The model under review builds one solid part; all positions refer to its coordinate system, in mm. Face numbers are marked on the shaded views. A direction names the side the tool comes from. Coordinates: 2 decimals unless noted, no trailing zeros. Write each loop counter-clockwise with the first axis right and the second up, starting at its lowest first coordinate (ties: lowest second). Pieces come first, ordered by that corner, then holes.
1) Add section A-A, the plane x = -8.5. State the section outline as (y, z) points.
2) For P1, Ø4, axis at x = 2.93, z = -7.36, coming from the +Y side; P2, Ø4, axis at x = -7.5, y = 6, coming from the +Z side; P3, Ø2, axis at x = -25, z = 10, coming from the +Y side; P4, Ø2, axis at x = -27.07, z = 22.64, coming from the -Y side, all flat-tipped, find the tip position at first contact; note any pin that passes through.
3) Add section C-C, the plane y = 1.5. State the section outline as (x, z) points.
4) For line 1 (Z direction, x = -21, y = 9.25); line 2 (Y direction, x = -29, z = 24); line 3 (Y direction, x = -18.5, z = 6), list the stretches that pass through material, from the lowest coordinate up.
5) Machinability: for the marked faces 1, 2, 3, 4 and 5, which of the approach directions +Z, -Z, +X, -X, +Y, -Y give a long, thin tool a straight path to every point of the face, cutting with its end or side? Answer none if there is none.
6) Add section D-D, the plane y = 13.25. State the section outline as (x, z) points.
7) Add section B-B, the plane x = -1.5. State the section outline as (y, z) points, then the cut area to 3 significant figures.
8) Mouldability with a two-part tool opening along Z and no side actions: class the marked faces 6, 7 and 8 as released by +Z, released by -Z, zero draft, split by the parting line, or undercut.
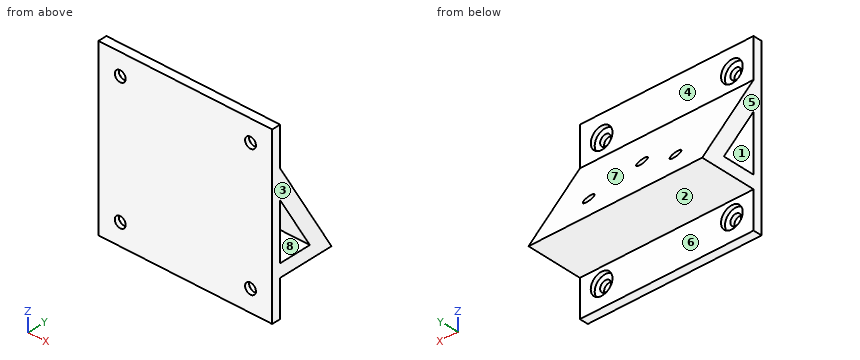
from build123d import *

# Parameters (mm, degrees)
SKETCH1_W           = 40
SKETCH1_H           = 40
BOSS_EXTRUDE1_DEPTH = 2
SKETCH2_R           = 1.25
CUT_EXTRUDE1_DEPTH  = 3
BOSS_EXTRUDE2_DEPTH = 40
SKETCH5_R           = 2.5
CUT_EXTRUDE3_DEPTH  = 1
CUT_EXTRUDE4_DEPTH  = 41
CUT_EXTRUDE5_REACH  = 19.232
SKETCH6_R           = 1.25
SKETCH11_R          = 2.6
CUT_EXTRUDE6_DEPTH  = 1.2


with BuildPart() as part:
    # Sketch1 → Boss-Extrude1 (new body)
    with BuildSketch(Plane(origin=(0, 0, 0), x_dir=(1, 0, 0), z_dir=(0, 1, 0))):
        with Locations((-12.069207341, -7.637914169)):
            Rectangle(SKETCH1_W, SKETCH1_H)
    extrude(amount=BOSS_EXTRUDE1_DEPTH)

    # Sketch2 → Cut-Extrude1 (cut, through all)
    with BuildSketch(Plane(origin=(0, 2, 0), x_dir=(1, 0, 0), z_dir=(0, 1, 0))):
        with Locations((-27.069207341, -22.637914169)):
            Circle(SKETCH2_R)
        with Locations((-27.069207341, 7.362085831)):
            Circle(SKETCH2_R)
        with Locations((2.930792659, 7.362085831)):
            Circle(SKETCH2_R)
        with Locations((2.930792659, -22.637914169)):
            Circle(SKETCH2_R)
    extrude(amount=-CUT_EXTRUDE1_DEPTH, mode=Mode.SUBTRACT)

    # Sketch4 → Boss-Extrude2 (add)
    with BuildSketch(Plane(origin=(7.930792659, 0, 0), x_dir=(0, 0, -1), z_dir=(1, 0, 0))):
        Polygon((-18.637914169, 2), (3.878746329, 2), (3.878746329, 15), align=None)
    extrude(amount=-BOSS_EXTRUDE2_DEPTH)

    # Sketch5 → Cut-Extrude3 (cut)
    with BuildSketch(Plane(origin=(0, 2, 0), x_dir=(1, 0, 0), z_dir=(0, 1, 0))):
        with Locations((2.930792659, 7.362085831)):
            Circle(SKETCH5_R)
        with Locations((2.930792659, -22.637914169)):
            Circle(SKETCH5_R)
        with Locations((37.902040206, 5.850032714)):
            Circle(SKETCH5_R)
        with Locations((-27.069207341, 7.362085831)):
            Circle(SKETCH5_R)
        with Locations((-27.069207341, -22.637914169)):
            Circle(SKETCH5_R)
    extrude(amount=-CUT_EXTRUDE3_DEPTH, mode=Mode.SUBTRACT)

    # Sketch9 → Cut-Extrude4 (cut, through all)
    with BuildSketch(Plane(origin=(7.930792659, 0, 0), x_dir=(0, 0, -1), z_dir=(1, 0, 0))):
        Polygon((-12.121253671, 2), (0.878746329, 2), (0.878746329, 9.505553499), align=None)
    extrude(amount=-CUT_EXTRUDE4_DEPTH, mode=Mode.SUBTRACT)

    # Sketch6 → Cut-Extrude5 (cut, up to next)
    with BuildSketch(Plane(origin=(0, 9.570453572, 5.525503946), x_dir=(1, 0, 0), z_dir=(0, 0.866025404, 0.5)), mode=Mode.PRIVATE) as cut_extrude5_sk1:
        with Locations((-22.069207341, 2.359092856)):
            Circle(SKETCH6_R)
    cut_extrude5_tool1 = extrude(cut_extrude5_sk1.sketch, amount=-CUT_EXTRUDE5_REACH, mode=Mode.PRIVATE) & part.part
    add(cut_extrude5_tool1.solids().sort_by_distance((-22.069207, 10.75, 3.48247))[0], mode=Mode.SUBTRACT)
    # Sketch6 → Cut-Extrude5 (cut, up to next)
    with BuildSketch(Plane(origin=(0, 9.570453572, 5.525503946), x_dir=(1, 0, 0), z_dir=(0, 0.866025404, 0.5)), mode=Mode.PRIVATE) as cut_extrude5_sk2:
        with Locations((-12.069207341, -2.640907144)):
            Circle(SKETCH6_R)
    cut_extrude5_tool2 = extrude(cut_extrude5_sk2.sketch, amount=-CUT_EXTRUDE5_REACH, mode=Mode.PRIVATE) & part.part
    add(cut_extrude5_tool2.solids().sort_by_distance((-12.069207, 8.25, 7.812597))[0], mode=Mode.SUBTRACT)
    # Sketch6 → Cut-Extrude5 (cut, up to next)
    with BuildSketch(Plane(origin=(0, 9.570453572, 5.525503946), x_dir=(1, 0, 0), z_dir=(0, 0.866025404, 0.5)), mode=Mode.PRIVATE) as cut_extrude5_sk3:
        with Locations((-2.069207341, 2.359092856)):
            Circle(SKETCH6_R)
    cut_extrude5_tool3 = extrude(cut_extrude5_sk3.sketch, amount=-CUT_EXTRUDE5_REACH, mode=Mode.PRIVATE) & part.part
    add(cut_extrude5_tool3.solids().sort_by_distance((-2.069207, 10.75, 3.48247))[0], mode=Mode.SUBTRACT)

    # Sketch11 → Cut-Extrude6 (cut)
    with BuildSketch(Plane(origin=(0, 6.748656802, 3.896338821), x_dir=(-1, 0, 0), z_dir=(0, -0.866025404, -0.5))):
        with Locations((2.069207341, 2.359092856)):
            Circle(SKETCH11_R)
        with Locations((22.069207341, 2.359092856)):
            Circle(SKETCH11_R)
        with Locations((12.069207341, -2.640907144)):
            Circle(SKETCH11_R)
    extrude(amount=-CUT_EXTRUDE6_DEPTH, mode=Mode.SUBTRACT)


solid = part.part
Geometry results:
1. outline: (0, -12.36) - (2, -12.36) - (2, -3.88) - (15, -3.88) - (2, 18.64) - (2, 27.64) - (0, 27.64) - close; hole (2, -0.88) - (9.51, -0.88) - (2, 12.12) - close
2. P1: stops at y = 1
2. P2: stops at z = 15.17
2. P3: stops at y = 7.56
2. P4: passes through
3. outline: (-32.07, -12.36) - (7.93, -12.36) - (7.93, 27.64) - (-32.07, 27.64) - close; hole circle Ø5 at (-27.07, -7.36); hole circle Ø5 at (-27.07, 22.64); hole circle Ø5 at (2.93, -7.36); hole circle Ø5 at (2.93, 22.64)
4. line 1: z = -3.88 to -0.88, -0.44 to -0.12, 3.36 to 6.08
4. line 2: y = 0 to 1
4. line 3: y = 0 to 2, 5.53 to 9.3
5. face 1: +X, -X
5. face 2: -Z, +X, -X, +Y
5. face 3: +Z, -Z, +X, +Y, -Y
5. face 4: +Z, +X, -X, +Y
5. face 5: +Z, -Z, -X, +Y, -Y
6. outline: (-32.07, -3.88) - (7.93, -3.88) - (7.93, -0.85) - (-32.07, -0.85) - close
7. outline: (0, -12.36) - (2, -12.36) - (2, -3.88) - (15, -3.88) - (11.31, 2.52) - (9.52, 1.49) - (10.24, 0.26) - (9.2, -0.34) - (9.51, -0.88) - (2, -0.88) - (2, 12.12) - (6.66, 4.05) - (7.7, 4.65) - (8.41, 3.42) - (10.19, 4.45) - (2, 18.64) - (2, 27.64) - (0, 27.64) - close
7. area: 167 mm2
8. face 6: zero draft
8. face 7: released by +Z
8. face 8: undercut
